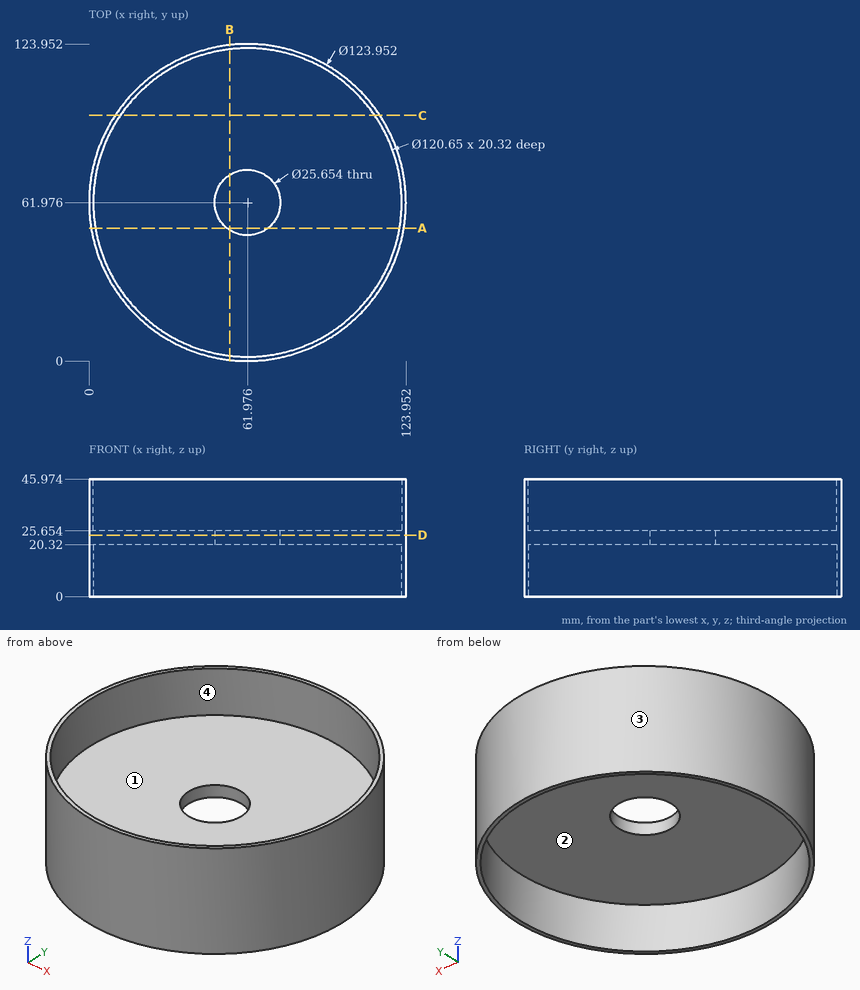
Could you check a few things on this drawing? It's one solid part, dimensions in mm from its lowest x, y, z. A direction names the side the tool comes from. Coordinates: 2 decimals unless noted, no trailing zeros. Order: outer loops, then holes, each group sorted by start corner. A loop starts at its lowest first (then second) coordinate and runs counter-clockwise, first axis right, second up. Notation, with made-up numbers: M 15.25,-23 L 69.25,-23 A22 ccw 69.25,-3 Z; hole C 67.25,10.25 d5. An arc over 180 degrees is marked long. Answer as a JSON object with one key per item and string values. Group by question number.
(1) For pin 1 (6 mm diameter, centred on x = 17, z = 38, fed in from -Y); pin 2 (1.5 mm diameter, centred on x = 18.5, z = 13.5, fed in from +Y); pin 3 (1.5 mm diameter, centred on x = 97.5, y = 73.5, fed in from +Z), each with a flat end and sliding along its axis, tell me the tip position at first contact or that it passes through.
(2) Suppose I cut it at A-A, the plane y = 52. Please give me the cut outline in (x, z).
(3) Suppose I cut it at D-D, the plane z = 24. Please give me the cut outline in (x, y).
(4) Which directions (+Z, -Z, +X, -X, +Y, -Y) give clear straight access to the entire face, cutting with the end or side of a thin tool? Please do the marked faces 1 and 2.
(5) Suppose I cut it at C-C, the plane y = 96. Please give me the cut outline in (x, z), then the cut area to 3 significant figures.
(6) Suppose I cut it at B-B, the plane x = 55. Please give me the cut outline in (y, z).
(7) I need wall thicknesses on probe 1 along Z at (x, y) = (54.5, 98); probe 2 along X at (y, z) = (80, 8.5); probe 3 along Y at (x, z) = (89, 34.5). Which ranges of each line are inside material? Lowest first, please.
(8) If we mould it in two halves opening along Y, with no side actions, what happens to the marked faces 3 and 4? For each: released by +Y, released by -Y, zero draft, split by the parting line, or undercut.
Values found:
{
 "1": {"pin 1": "stops at y = 16.38", "pin 2": "stops at y = 106.87", "pin 3": "stops at z = 25.65"},
 "2": {"outline": "M 0.81,0 L 2.48,0 L 2.48,20.32 L 53.91,20.32 L 53.91,25.65 L 2.48,25.65 L 2.48,45.97 L 0.81,45.97 Z; M 70.04,20.32 L 121.47,20.32 L 121.47,0 L 123.14,0 L 123.14,45.97 L 121.47,45.97 L 121.47,25.65 L 70.04,25.65 Z"},
 "3": {"outline": "C 61.98,61.98 d123.95; hole C 61.98,61.98 d25.65"},
 "4": {"face 1": "+Z", "face 2": "-Z"},
 "5": {"outline": "M 10.17,0 L 12.16,0 L 12.16,20.32 L 111.79,20.32 L 111.79,0 L 113.78,0 L 113.78,45.97 L 111.79,45.97 L 111.79,25.65 L 12.16,25.65 L 12.16,45.97 L 10.17,45.97 Z", "area": "714 mm^2"},
 "6": {"outline": "M 0.39,0 L 2.06,0 L 2.06,20.32 L 51.21,20.32 L 51.21,25.65 L 2.06,25.65 L 2.06,45.97 L 0.39,45.97 Z; M 72.74,20.32 L 121.9,20.32 L 121.9,0 L 123.56,0 L 123.56,45.97 L 121.9,45.97 L 121.9,25.65 L 72.74,25.65 Z"},
 "7": {"probe 1": "z = 20.32 to 25.65", "probe 2": "x = 2.68 to 4.41, 119.55 to 121.27", "probe 3": "y = 6.2 to 8.04, 115.91 to 117.75"},
 "8": {"face 3": "split by the parting line", "face 4": "undercut"}
}
